Build history of the part. All positions in model axes, mm. Face numbers are marked on the shaded views. A direction names the side the tool comes from. Give positions to 0.01 mm unless a question says otherwise; leave off trailing zeros. Order: outer loops, then holes, each group sorted by start corner. A loop starts at its lowest first (then second) coordinate and runs counter-clockwise, first axis right, second up. Notation, with made-up numbers: M 5.25,-10.5 L 39.25,-10.5 A24 ccw 39.25,25.5 Z; hole C 58.25,-23 d9. An arc over 180 degrees is marked long. Answer as CSV lines item,"result".
from build123d import *

# Parameters (mm, degrees)
SKETCH1_W          = 133.35
SKETCH1_H          = 20.32
EXTRUDE1_DEPTH     = 63.5
CUT_EXTRUDE1_DEPTH = 21.32
FILLET1_R          = 6.35
CUT_EXTRUDE2_DEPTH = 64.5
SKETCH6_R          = 2.07645
CUT_EXTRUDE5_DEPTH = 67.675


with BuildPart() as part:
    # Sketch1 → Extrude1 (new body)
    with BuildSketch(Plane.XY):
        with Locations((0, 14.12875)):
            Rectangle(SKETCH1_W, SKETCH1_H)
    extrude(amount=EXTRUDE1_DEPTH)

    # Sketch2 → Cut-Extrude1 (cut, through all)
    with BuildSketch(Plane.XZ.offset(-3.96875)):
        with BuildLine():
            Line((-10.033, 23.761628021), (-10.033, 63.5))
            ThreePointArc((-10.033, 63.5), (-23.144173937, 58.069173937), (-28.575, 44.958))
            Line((-28.575, 44.958), (-28.575, 31.75))
            ThreePointArc((-28.575, 31.75), (-30.434871939, 27.259871939), (-34.925, 25.4))
            Line((-34.925, 25.4), (-66.675, 25.4))
            Line((-66.675, 25.4), (-66.675, 63.5))
            Line((-66.675, 63.5), (-66.675, 81.695932909))
            Line((-66.675, 81.695932909), (66.675, 81.695932909))
            Line((66.675, 81.695932909), (66.675, 63.5))
            Line((66.675, 63.5), (66.675, 25.4))
            Line((66.675, 25.4), (34.925, 25.4))
            ThreePointArc((34.925, 25.4), (30.434871939, 27.259871939), (28.575, 31.75))
            Line((28.575, 31.75), (28.575, 44.958))
            ThreePointArc((28.575, 44.958), (23.144173937, 58.069173937), (10.033, 63.5))
            Line((10.033, 63.5), (10.033, 23.761628021))
            ThreePointArc((10.033, 23.761628021), (0, 20.6), (-10.033, 23.761628021))
        make_face()
    extrude(amount=-CUT_EXTRUDE1_DEPTH, mode=Mode.SUBTRACT)

    # Fillet1
    fillet1_edges = [part.edges().sort_by_distance(p)[0] for p in [
        (-66.675, 14.12875, 25.4),
        (66.675, 14.12875, 25.4),
    ]]
    fillet(fillet1_edges, radius=FILLET1_R)

    # Sketch3 → Cut-Extrude2 (cut, through all)
    with BuildSketch(Plane(origin=(0, 0, 0), x_dir=(-1, 0, 0), z_dir=(0, 0, -1))):
        with BuildLine():
            Line((-52.3875, 18.89125), (-42.8625, 18.89125))
            ThreePointArc((-42.8625, 18.89125), (-38.1, 14.12875), (-42.8625, 9.36625))
            Line((-42.8625, 9.36625), (-52.3875, 9.36625))
            ThreePointArc((-52.3875, 9.36625), (-57.15, 14.12875), (-52.3875, 18.89125))
        make_face()
        with BuildLine():
            Line((52.3875, 9.36625), (42.8625, 9.36625))
            ThreePointArc((42.8625, 9.36625), (38.1, 14.12875), (42.8625, 18.89125))
            Line((42.8625, 18.89125), (52.3875, 18.89125))
            ThreePointArc((52.3875, 18.89125), (57.15, 14.12875), (52.3875, 9.36625))
        make_face()
    extrude(amount=-CUT_EXTRUDE2_DEPTH, mode=Mode.SUBTRACT)

    # Sketch6 → Cut-Extrude5 (cut, through all)
    with BuildSketch(Plane(origin=(0, 0, 0), x_dir=(0, 0, -1), z_dir=(1, 0, 0))):
        with Locations((-38.1, 14.12875)):
            Circle(SKETCH6_R)
    extrude(amount=CUT_EXTRUDE5_DEPTH, mode=Mode.SUBTRACT)


solid = part.part
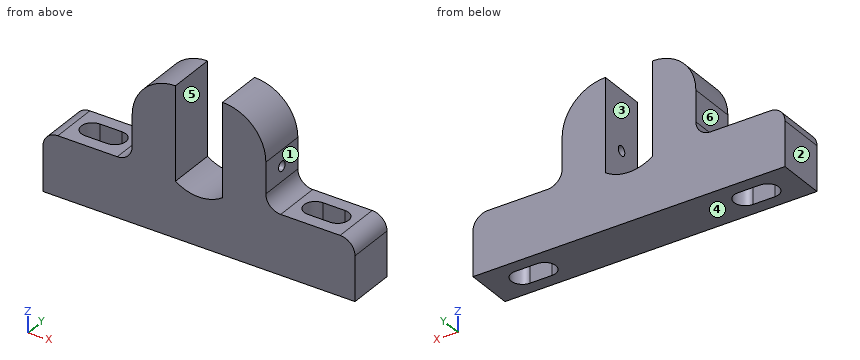
Item 1: Drop flat-ended pins along their axis: pin 1 (4 mm diameter, centred on y = 10.5, z = 36, fed in from -X) (3 decimals); pin 2 (1 mm diameter, centred on x = -14.5, y = 12.5, fed in from +Z); pin 3 (2 mm diameter, centred on x = 48, y = 10, fed in from +Z). Give the stop position or say it passes through.
Geometry says:
pin 1,"stops at x = -28.575"
pin 2,"stops at z = 63.07"
pin 3,"stops at z = 25.4"
Item 2: Band-saw the part on D-D (y = 7.5). Give the cut face in (x, z) (3 decimals).
Geometry says:
outline,"M -66.675,0 L 66.675,0 L 66.675,19.05 A6.35 ccw 60.325,25.4 L 34.925,25.4 A6.35 cw 28.575,31.75 L 28.575,44.958 A18.542 ccw 10.033,63.5 L 10.033,23.762 A17.5 cw -10.033,23.762 L -10.033,63.5 A18.542 ccw -28.575,44.958 L -28.575,31.75 A6.35 cw -34.925,25.4 L -60.325,25.4 A6.35 ccw -66.675,19.05 Z"
Item 3: Pull direction X, two halves, no side cores. Call the marked faces 1, 2 and 3: released by +X, released by -X, zero draft, split by the parting line, or undercut.
Geometry says:
face 1,"released by +X"
face 2,"released by -X"
face 3,"undercut"
Item 4: Band-saw the part on C-C (z = 28). Give the cut face in (x, y), and give its area (3 significant figures).
Geometry says:
outline,"M -29.8,3.97 L -10.03,3.97 L -10.03,24.29 L -29.8,24.29 Z; M 10.03,3.97 L 29.8,3.97 L 29.8,24.29 L 10.03,24.29 Z"
area,"803 mm2"
Item 5: 3-axis set-ups, long thin cutter, end or side, ignore diameter. For the marked faces 4, 5 and 6: which of +Z, -Z, +X, -X, +Y, -Y reach the whole face in a straight line?
Geometry says:
face 4,"-Z, +X, -X, +Y, -Y"
face 5,"+Z, +Y, -Y"
face 6,"+Z, -X, +Y, -Y"
Item 6: Probe line 1 along Y through (x, z) = (21.25, 38.1); line 2 along X through (y, z) = (7, 42.5) (3 decimals); line 3 along Z through (x, y) = (58.5, 14.25). List the from-to ranges inside material, lowest first. Write a range as from..to.
Geometry says:
line 1,"y = 3.97..12.05, 16.21..24.29"
line 2,"x = -28.575..-10.033, 10.033..28.575"
line 3,"z = 0..25.4"
Item 7: Band-saw the part on B-B (x = -51). Give the cut face in (y, z).
Geometry says:
outline,"M 3.97,0 L 9.37,0 L 9.37,25.4 L 3.97,25.4 Z; M 18.89,0 L 24.29,0 L 24.29,25.4 L 18.89,25.4 Z"
Item 8: Band-saw the part on A-A (z = 38.1). Give the cut face in (x, y) (3 decimals).
Geometry says:
outline,"M -28.575,3.969 L -10.033,3.969 L -10.033,24.289 L -28.575,24.289 Z; M 10.033,3.969 L 28.575,3.969 L 28.575,12.052 L 10.033,12.052 Z; M 10.033,16.205 L 28.575,16.205 L 28.575,24.289 L 10.033,24.289 Z"
